Solid Edge part; units mm, degrees
sketch "Sketch1" plane through (0, 0, 0) normal (0, 0, 1) x (1, 0, 0)
  line L0 (11.7678, 8.2322) -> (1.7678, -1.7678)
  line L1 (1.7678, -1.7678) -> (1.7678, 5.3033)
  line L2 (1.7678, 5.3033) -> (6.4645, 10)
  line L3 (6.4645, 10) -> (-1.0355, 17.5)
  line L4 (-1.0355, 17.5) -> (-11.7678, 17.5)
  line L5 (-11.7678, 17.5) -> (-11.7678, 22.5)
  line L6 (-11.7678, 22.5) -> (0, 22.5)
  arc A0 (1.7678, 21.7678) -> (0, 22.5) centre (0, 20) ccw
  line L7 (1.7678, 21.7678) -> (11.7678, 11.7678)
  line L8 (11.7678, 11.7678) -> (11.7678, 8.2322)
  circle A1 centre (-9.1161, 20.0115) radius 1
extrude "ExtrudedProtrusion_1" add sketch "Sketch1" along normal blind 2
sketch "Sketch2" plane through (0, 0, 0) normal (0, 0, 1) x (1, 0, 0)
  circle A0 centre (-9.1161, 10) radius 1
  line L0 (-1.7678, 21.7678) -> (-11.7678, 11.7678)
  line L1 (-11.7678, 11.7678) -> (-11.7678, 8.2322)
  line L2 (-11.7678, 8.2322) -> (-1.7678, -1.7678)
  line L3 (-1.7678, -1.7678) -> (-1.7678, 5.3033)
  line L4 (-1.7678, 5.3033) -> (-6.4645, 10)
  line L5 (-6.4645, 10) -> (1.7678, 18.2322)
  arc A1 (-1.7678, 21.7678) -> (1.7678, 18.2322) centre (0, 20) cw
  arc A2 (-1.7678, 21.7678) -> (1.7678, 18.2322) centre (0, 20) cw
  arc A3 (-1.7678, 21.7678) -> (1.7678, 18.2322) centre (0, 20) cw
extrude "ExtrudedProtrusion_2" add sketch "Sketch2" against normal blind 2
hole "Hole_1" at (0, 20, -2) direction (0, 0, 1) diameter 2 end up to next
Could you check a few things on this model? Use its own coordinates, in mm. A direction names the side the tool comes from. Round coordinates to 2 decimals unless told otherwise and drop trailing zeros. Loops run counter-clockwise (first coordinate to the right, second up) from the corner with the lowest first, then second, coordinate; pieces in that order, holes last. Notation, with made-up numbers: (25, 34.25) -> (32, 34.25) arc R23 ccw to (32, 44.25) -> close; hole circle Ø1 at (-10, 87.5). An arc over 180 degrees is marked (long way). Put each result on its own line as item: value.
Q1. Please list where these lines run through material, in increasing order: line 1 (Z direction, x = -1.25, y = 16); line 2 (Y direction, x = -4, z = -0.15); line 3 (X direction, y = 20, z = 0.3). Write a range as from..to.
Checks:
line 1: -2..0
line 2: 0.46..7.54, 12.46..19.54
line 3: -11.77..-10.12, -8.12..-1, 1..3.54
Q2. For pin 1 Ø1.6 at (x, z) = (-5, 1) entering from -Y; pin 2 Ø1 at (y, z) = (2, 1) entering from -X; pin 3 Ø1 at (y, z) = (2.5, -1) entering from +X, each with a flat end and sliding along its axis, tell me the tip position at first contact or that it passes through.
Checks:
pin 1: y = 17.5
pin 2: x = 1.77
pin 3: x = -1.77
Q3. I want a section at B-B on y = 0. Write out the boundary of the cut face in (x, z).
Checks:
outline: (-3.54, -2) -> (-1.77, -2) -> (-1.77, 0) -> (-3.54, 0) -> close; (1.77, 0) -> (3.54, 0) -> (3.54, 2) -> (1.77, 2) -> close
Q4. I want a section at A-A on z = -0.75. Write out the boundary of the cut face in (x, y), and give its area (3 significant figures).
Checks:
outline: (-11.77, 8.23) -> (-1.77, -1.77) -> (-1.77, 5.3) -> (-6.46, 10) -> (1.77, 18.23) arc R2.5 ccw to (-1.77, 21.77) -> (-11.77, 11.77) -> close; hole circle Ø2 at (-9.12, 10); hole circle Ø2 at (0, 20)
area: 129 mm2
Q5. Thinking about a two-plate mould opening in Y: for faces 1 (the flat face through (-1.768, 2, -1)), 2 (the cylindrical face through (1.806, 21.728, -0.861)), 3 (the flat face through (4.083, 7.619, 0.986)), which applies, pulls with the +Y half, pulls with the -Y half, needs draft (parallel to the pull), parting line crosses it, or undercut?
Checks:
face 1: needs draft
face 2: parting line crosses it
face 3: undercut
Q6. I want a section at D-D on z = 0.8. Write out the boundary of the cut face in (x, y).
Checks:
outline: (-11.77, 17.5) -> (-1.04, 17.5) -> (6.46, 10) -> (1.77, 5.3) -> (1.77, -1.77) -> (11.77, 8.23) -> (11.77, 11.77) -> (1.77, 21.77) arc R2.5 ccw to (0, 22.5) -> (-11.77, 22.5) -> close; hole circle Ø2 at (-9.12, 20.01); hole circle Ø2 at (0, 20)
Q7. I want a section at C-C on x = -9.75. Write out the boundary of the cut face in (y, z), and give its area (3 significant figures).
Checks:
outline: (6.21, -2) -> (9.23, -2) -> (9.23, 0) -> (6.21, 0) -> close; (10.77, -2) -> (13.79, -2) -> (13.79, 0) -> (10.77, 0) -> close; (17.5, 0) -> (19.24, 0) -> (19.24, 2) -> (17.5, 2) -> close; (20.78, 0) -> (22.5, 0) -> (22.5, 2) -> (20.78, 2) -> close
area: 19.0 mm2
Q8. Which directions (+Z, -Z, +X, -X, +Y, -Y) give clear straight access to the entire face, cutting with the end or side of a thin tool? Please do faces 4 (the flat face through (-7, 21, 0)), 5 (the flat face through (-2.406, 14.058, -0.986)), 6 (the flat face through (-6, 8, 0)).
Checks:
face 4: -Z, -X, +Y
face 5: -Z, +X
face 6: +Z, -X, -Y
